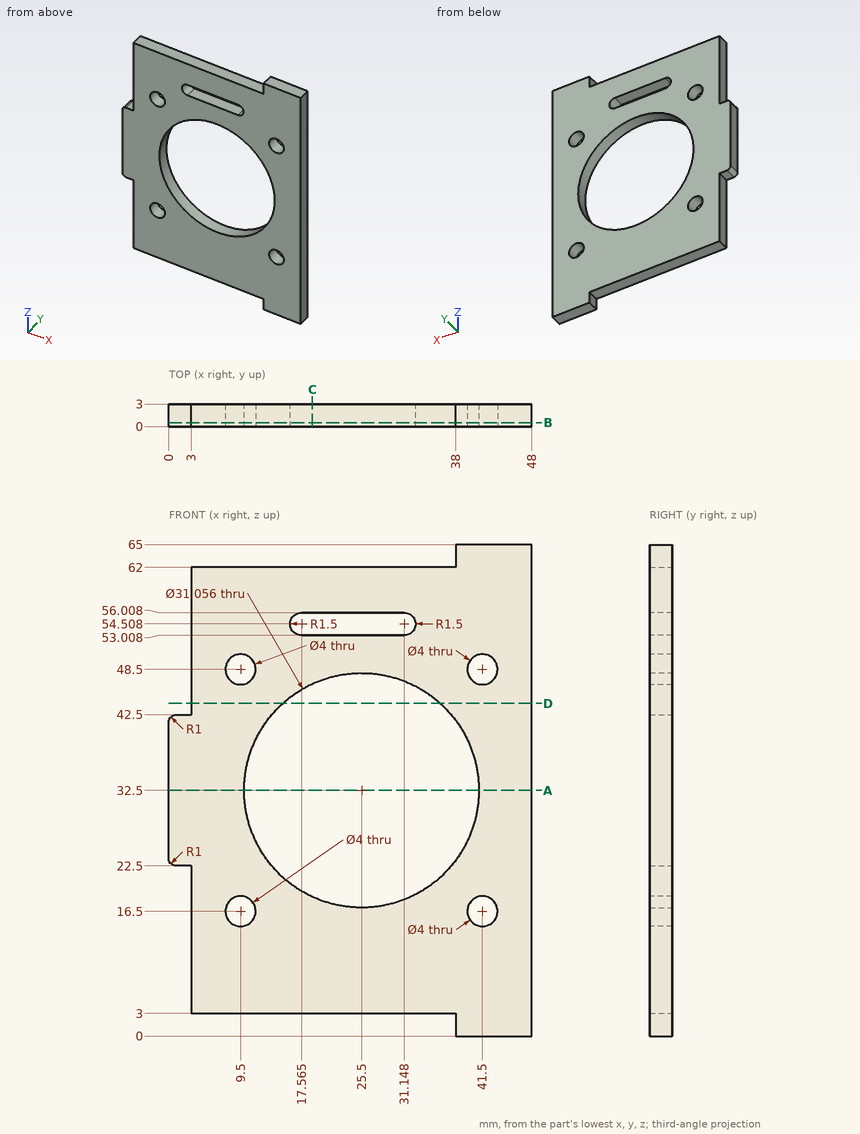
Job drawing, mm, ordinate dimensions from the low corner. One solid piece. Round coordinates to 2 decimals unless told otherwise and drop trailing zeros. Loops run counter-clockwise (first coordinate to the right, second up) from the corner with the lowest first, then second, coordinate; pieces in that order, holes last. Notation, with made-up numbers: M 31.25,3 L 39.25,3 A22 cw 39.25,16 Z; hole C -22,38 d4. An arc over 180 degrees is marked long. Answer as CSV lines item,"result".
1. Cut at B-B on y = 0.55. Write the cut outline in (x, z) (1 decimal).
Resolved:
outline,"M 0,23.5 A1 ccw 1,22.5 L 3,22.5 L 3,3 L 38,3 L 38,0 L 48,0 L 48,65 L 38,65 L 38,62 L 3,62 L 3,42.5 L 1,42.5 A1 ccw 0,41.5 Z; hole C 9.5,16.5 d4; hole C 9.5,48.5 d4; hole C 25.5,32.5 d31.1; hole M 17.6,53 L 31.1,53 A1.5 ccw 31.1,56 L 17.6,56 A1.5 ccw Z; hole C 41.5,16.5 d4; hole C 41.5,48.5 d4"
2. Cut at A-A on z = 32.5. Write the cut outline in (x, y).
Resolved:
outline,"M 0,0 L 9.97,0 L 9.97,3 L 0,3 Z; M 41.03,0 L 48,0 L 48,3 L 41.03,3 Z"
3. Cut at D-D on z = 44. Write the cut outline in (x, y).
Resolved:
outline,"M 3,0 L 15.07,0 L 15.07,3 L 3,3 Z; M 35.93,0 L 48,0 L 48,3 L 35.93,3 Z"
4. Flat gauge pins, fed straight in: P1, Ø5, axis at x = 9.5, z = 16.5, coming from the -Y side; P2, Ø6, axis at x = 23.5, z = 44, coming from the +Y side; P3, Ø0.9, axis at y = 1, z = 14.5, coming from the -X side; P4, Ø1, axis at x = 2, y = 2, coming from the +Z side. Where does each tip first touch, or does it go through?
Resolved:
P1,"stops at y = 0"
P2,"passes through"
P3,"stops at x = 3"
P4,"stops at z = 42.5"
5. Cut at C-C on x = 19. Write the cut outline in (y, z).
Resolved:
outline,"M 0,3 L 3,3 L 3,18.4 L 0,18.4 Z; M 0,46.6 L 3,46.6 L 3,53.01 L 0,53.01 Z; M 0,56.01 L 3,56.01 L 3,62 L 0,62 Z"
6. Wall check: probe 1 along Z at (x, y) = (9.5, 2.2); probe 2 along X at (y, z) = (1.1, 16.5); probe 3 along Z at (x, y) = (41.5, 1.45). Give the ranges that are in metal, low to high. Write a range as [from, to].
Resolved:
probe 1,"z = [3, 14.5], [18.5, 46.5], [50.5, 62]"
probe 2,"x = [3, 7.5], [11.5, 39.5], [43.5, 48]"
probe 3,"z = [0, 14.5], [18.5, 46.5], [50.5, 65]"
